from build123d import *

# Parameters (mm, degrees)
SKETCH13_W         = 16
SKETCH13_H         = 3
CHAMFER1_SIZE      = 0.75
CUT_EXTRUDE2_DEPTH = 2.31


with BuildPart() as part:
    # Sketch13 → Revolve1 (revolve)
    with BuildSketch(Plane(origin=(0, 0, 0), x_dir=(0, 0, -1), z_dir=(1, 0, 0)), mode=Mode.PRIVATE) as revolve1_sk:
        with Locations((1.65, 1.5)):
            Rectangle(SKETCH13_W, SKETCH13_H)
    revolve(revolve1_sk.sketch.rotate(Axis((0, 0, 9.65), (0, 0, -1)), 90), axis=Axis((0, 0, 9.65), (0, 0, -1)))

    # Chamfer1
    chamfer1_edges = [part.edges().sort_by_distance(p)[0] for p in [
        (-3, 0, -9.65),
    ]]
    chamfer(chamfer1_edges, length=CHAMFER1_SIZE)

    # Sketch7 → Revolve2 (revolve)
    with BuildSketch(Plane(origin=(0, 0, 0), x_dir=(0, 0, -1), z_dir=(1, 0, 0)), mode=Mode.PRIVATE) as revolve2_sk:
        with BuildLine():
            Line((-6.35, 5.25), (-6.35, 0))
            Line((-6.35, 0), (-9.65, 0))
            Line((-9.65, 0), (-9.65, 3))
            ThreePointArc((-9.65, 3), (-8.577614941, 4.306626435), (-7.175, 5.25))
            Line((-7.175, 5.25), (-7.175, 6.8))
            Line((-7.175, 6.8), (-6.35, 6.8))
            Line((-6.35, 6.8), (-6.35, 5.25))
        make_face()
    revolve(revolve2_sk.sketch.rotate(Axis((0, 0, 9.65), (0, 0, -1)), 180), axis=Axis((0, 0, 9.65), (0, 0, -1)))

    # Sketch5 → Cut-Extrude2 (cut)
    with BuildSketch(Plane.XY.offset(9.65)):
        Polygon((2, -1.154700538), (2, 1.154700538), (0, 2.309401077), (-2, 1.154700538), (-2, -1.154700538), (0, -2.309401077), align=None)
    extrude(amount=-CUT_EXTRUDE2_DEPTH, mode=Mode.SUBTRACT)

    # Cut-Extrude3 cone 1 section (through the dimple's axis) → Cut-Extrude3 (revolve, cut)
    with BuildSketch(Plane(origin=(0, 0, 9.65), x_dir=(0, -1, 0), z_dir=(1, 0, 0))):
        Polygon((0, 0), (2.309401077, 0), (0, 2.309401077), align=None)
    revolve(axis=Axis((0, 0, 9.65), (0, 0, -1)), mode=Mode.SUBTRACT)


solid = part.part
The model under review builds one solid part; all positions refer to its coordinate system, in mm. A direction names the side the tool comes from. Give positions to 0.01 mm unless a question says otherwise; leave off trailing zeros. Order: outer loops, then holes, each group sorted by start corner. A loop starts at its lowest first (then second) coordinate and runs counter-clockwise, first axis right, second up. Notation, with made-up numbers: (-15, -35.5) -> (6, -35.5) arc R20 ccw to (6, -17.5) -> close; hole circle Ø1 at (-19.75, -21.75). An arc over 180 degrees is marked (long way). Write item = value, one per line. Start each with the question number.
(1) For L1, parallel to Z at x = 5.5, y = 3.5 (3 decimals); L2, parallel to Z at x = 1.25, y = -1.25; L3, parallel to Y at x = 2, z = -4.75, list the stretches that pass through material, from the lowest coordinate up. Write a range as from..to.
(2) For pin 1 Ø4 at (y, z) = (3, 3) entering from +X; pin 2 Ø2 at (x, y) = (0, -0.5) entering from +Z; pin 3 Ø3 at (y, z) = (3, 5.5) entering from +X, all flat-tipped, find the tip position at first contact; note any pin that passes through.
(3) Take a section at B-B (z = -1.5). Write out the cut boundary in (x, y).
(4) Draft analysis for pull direction X (two halves, no side actions). For faces 4 (the flat face through (5, 3, 7.175)), 5 (the cylindrical face through (6.64, 1.47, 6.76)), 6 (the conical face through (-1.06, -1.87, 9.49)), state which applies: +X half, -X half, draft (parallel to the pull), parting line (faces both ways), or undercut.
(5) Tool access review of faces 1 (the flat face through (1, -3, 6.35)), 2 (the flat face through (2, 2, 9.65)), 3 (the flat face through (-2, 0, 9)): name each direction out of +Z, -Z, +X, -X, +Y, -Y from which nothing blocks a thin tool from reaching the whole face with its end or side.
Returned:
q1.L1 = 6.35..7.175
q1.L2 = -9.65..7.34
q1.L3 = -2.24..2.24
q2.pin_1 = 2.83
q2.pin_2 = 7.34
q2.pin_3 = 6.57
q3.outline = circle Ø6 at (0, 0)
q4.face_4 = draft
q4.face_5 = parting line
q4.face_6 = undercut
q5.face_1 = -Z
q5.face_2 = +Z, +X, -X, +Y, -Y
q5.face_3 = +Z
